Geometry: final body of the model. Coordinates: model frame, mm. A direction names the side the tool comes from. Round coordinates to 2 decimals unless told otherwise and drop trailing zeros. Write each loop counter-clockwise with the first axis right and the second up, starting at its lowest first coordinate (ties: lowest second). Pieces come first, ordered by that corner, then holes.
from build123d import *

# Parameters (mm, degrees)
PAD_DEPTH       = 1.6
SKETCH001_W     = 66
SKETCH001_H     = 48
PAD001_DEPTH    = 26.6
PAD002_DEPTH    = 11.2
SKETCH003_W     = 16
SKETCH003_H     = 8
POCKET_DEPTH    = 16
SKETCH005_R     = 4
SKETCH005_R_2   = 2
PAD003_DEPTH    = 15.6
SKETCH006_W     = 1
SKETCH006_H     = 34.5
SKETCH006_H_2   = 12
PAD004_DEPTH    = 11.6
SKETCH007_R     = 4
SKETCH007_R_2   = 2
PAD005_DEPTH    = 11.6
PAD006_DEPTH    = 24
PAD007_DEPTH    = 66
POCKET002_DEPTH = 0.6
SKETCH018_W     = 48
SKETCH018_H     = 7.5
POCKET003_DEPTH = 2.5
SKETCH008_R     = 1.4
POCKET004_DEPTH = 8


with BuildPart() as part:
    # Sketch → Pad (new body)
    with BuildSketch(Plane.XY):
        with BuildLine():
            Line((-36, 28), (36, 28))
            ThreePointArc((37, 27), (36.707107, 27.707107), (36, 28))
            Line((37, 27), (37, -27))
            ThreePointArc((36, -28), (36.707107, -27.707107), (37, -27))
            Line((36, -28), (-36, -28))
            ThreePointArc((-37, -27), (-36.707107, -27.707107), (-36, -28))
            Line((-37, -27), (-37, 27))
            ThreePointArc((-36, 28), (-36.707107, 27.707107), (-37, 27))
        make_face()
        with BuildLine():
            ThreePointArc((-12.5, 5), (-17.5, 0), (-12.5, -5))
            Line((-12.5, -5), (12.5, -5))
            ThreePointArc((12.5, -5), (17.5, 0), (12.5, 5))
            Line((12.5, 5), (-12.5, 5))
        make_face(mode=Mode.SUBTRACT)
    extrude(amount=PAD_DEPTH)

    # Sketch001 → Pad001 (join)
    with BuildSketch(Plane.XY):
        with BuildLine():
            Line((-36, 28), (36, 28))
            ThreePointArc((37, 27), (36.707107, 27.707107), (36, 28))
            Line((37, 27), (37, -27))
            ThreePointArc((36, -28), (36.707107, -27.707107), (37, -27))
            Line((36, -28), (-36, -28))
            ThreePointArc((-37, -27), (-36.707107, -27.707107), (-36, -28))
            Line((-37, -27), (-37, 27))
            ThreePointArc((-36, 28), (-36.707107, 27.707107), (-37, 27))
        make_face()
        Rectangle(SKETCH001_W, SKETCH001_H, mode=Mode.SUBTRACT)
    extrude(amount=PAD001_DEPTH)

    # Sketch002 → Pad002 (join)
    with BuildSketch(Plane.XY):
        with BuildLine():
            Line((51.5, 9.499999), (38.5, 9.499999))
            ThreePointArc((37, 11.000001), (37.439339, 9.93934), (38.5, 9.499999))
            Line((37, 11.000001), (37, 0))
            Line((37, 0), (37, -11.000001))
            ThreePointArc((38.5, -9.500001), (37.43934, -9.939341), (37, -11.000001))
            Line((38.5, -9.500001), (51.5, -9.500001))
            ThreePointArc((51.5, -9.500001), (52.56066, -9.060661), (53, -8.000001))
            Line((53, 7.999999), (53, -8.000001))
            ThreePointArc((53, 7.999999), (52.56066, 9.060659), (51.5, 9.499999))
        make_face()
    extrude(amount=PAD002_DEPTH)

    # Sketch003 (on DatumPlane) → Pocket (cut)
    with BuildSketch(Plane.YZ.offset(33)):
        with Locations((0, 5.6)):
            Rectangle(SKETCH003_W, SKETCH003_H)
    extrude(amount=POCKET_DEPTH, mode=Mode.SUBTRACT)

    # Sketch005 → Pad003 (join)
    with BuildSketch(Plane.XY):
        with Locations((-11, 15)):
            Circle(SKETCH005_R)
        with Locations((-11, 15)):
            Circle(SKETCH005_R_2, mode=Mode.SUBTRACT)
        with Locations((11, 15)):
            Circle(SKETCH005_R)
        with Locations((11, 15)):
            Circle(SKETCH005_R_2, mode=Mode.SUBTRACT)
    extrude(amount=PAD003_DEPTH)

    # Sketch006 → Pad004 (join)
    with BuildSketch(Plane.XY):
        with Locations((-31, -6.75)):
            Rectangle(SKETCH006_W, SKETCH006_H)
        with Locations((29, -18)):
            Rectangle(SKETCH006_W, SKETCH006_H_2)
    extrude(amount=PAD004_DEPTH)

    # Sketch007 → Pad005 (join)
    with BuildSketch(Plane.XY):
        with Locations((-24, 15)):
            Circle(SKETCH007_R)
        with Locations((-24, 15)):
            Circle(SKETCH007_R_2, mode=Mode.SUBTRACT)
        with Locations((24, 15)):
            Circle(SKETCH007_R)
        with Locations((24, 15)):
            Circle(SKETCH007_R_2, mode=Mode.SUBTRACT)
    extrude(amount=PAD005_DEPTH)

    # Sketch009 → Pad006 (join, symmetric)
    with BuildSketch(Plane.XZ):
        Polygon((-33, 26.6), (-29, 26.6), (-29, 23.6), (-33, 18.832986), align=None)
        Polygon((29, 26.6), (33, 26.6), (33, 18.832986), (29, 23.6), align=None)
    extrude(amount=PAD006_DEPTH, both=True)

    # Sketch010 (on DatumPlane) → Pad007 (join)
    with BuildSketch(Plane(origin=(-33, 0, 0), x_dir=(0, -1, 0), z_dir=(-1, 0, 0))):
        Polygon((-24, 18.832986), (-20, 23.6), (-20, 26.6), (-24, 26.6), align=None)
        Polygon((24, 26.6), (20, 26.6), (20, 23.6), (24, 18.832986), align=None)
    extrude(amount=-PAD007_DEPTH)

    # Sketch011 (on DatumPlane) → Pocket002 (cut)
    with BuildSketch(Plane.XY.offset(26.6)):
        with BuildLine():
            Line((-27.75, 22.25), (27.75, 22.25))
            ThreePointArc((31.25, 18.75), (30.224874, 21.224874), (27.75, 22.25))
            Line((31.25, 18.75), (31.25, -18.75))
            ThreePointArc((27.75, -22.25), (30.224874, -21.224874), (31.25, -18.75))
            Line((27.75, -22.25), (-27.75, -22.25))
            ThreePointArc((-31.25, -18.75), (-30.224874, -21.224874), (-27.75, -22.25))
            Line((-31.25, -18.75), (-31.25, 18.75))
            ThreePointArc((-27.75, 22.25), (-30.224874, 21.224874), (-31.25, 18.75))
        make_face()
        with BuildLine():
            Line((-27.75, 21.25), (27.75, 21.25))
            ThreePointArc((30.25, 18.75), (29.517767, 20.517767), (27.75, 21.25))
            Line((30.25, 18.75), (30.25, -18.75))
            ThreePointArc((27.75, -21.25), (29.517767, -20.517767), (30.25, -18.75))
            Line((27.75, -21.25), (-27.75, -21.25))
            ThreePointArc((-30.25, -18.75), (-29.517767, -20.517767), (-27.75, -21.25))
            Line((-30.25, -18.75), (-30.25, 18.75))
            ThreePointArc((-27.75, 21.25), (-29.517767, 20.517767), (-30.25, 18.75))
        make_face(mode=Mode.SUBTRACT)
    extrude(amount=-POCKET002_DEPTH, mode=Mode.SUBTRACT)

    # Sketch018 (on DatumPlane) → Pocket003 (cut)
    with BuildSketch(Plane(origin=(-33, 0, 0), x_dir=(0, -1, 0), z_dir=(-1, 0, 0))):
        with Locations((0, 5.35)):
            Rectangle(SKETCH018_W, SKETCH018_H)
    extrude(amount=POCKET003_DEPTH, mode=Mode.SUBTRACT)

    # Sketch008 (on DatumPlane) → Pocket004 (cut)
    with BuildSketch(Plane.XY.offset(26.6)):
        with Locations((-34, 25)):
            Circle(SKETCH008_R)
        with Locations((0, 25)):
            Circle(SKETCH008_R)
        with Locations((34, 25)):
            Circle(SKETCH008_R)
        with Locations((-34, -25)):
            Circle(SKETCH008_R)
        with Locations((0, -25)):
            Circle(SKETCH008_R)
        with Locations((34, -25)):
            Circle(SKETCH008_R)
        with Locations((-34, 0)):
            Circle(SKETCH008_R)
        with Locations((34, 0)):
            Circle(SKETCH008_R)
    extrude(amount=-POCKET004_DEPTH, mode=Mode.SUBTRACT)


solid = part.part
1) Line query: probe 1 along Y at (x, z) = (-24, 5); probe 2 along Y at (x, z) = (0, 24.75); probe 3 along X at (y, z) = (-4.5, 5.25). Output: solid intervals per line, ascending.
2) Draft query along Y for faces 1 (the flat face through (37, 0, 13)), 2 (the flat face through (9, 14, 15.6)), 3 (the flat face through (45, 9.5, 6)). Return one class per face: pulls with the +Y half, pulls with the -Y half, needs draft (parallel to the pull), parting line crosses it, or undercut.
3) Reachability of faces 4 (the flat face through (-29.3, -0.1, 26.6)), 5 (the flat face through (0, 20, 25)), 6 (the flat face through (49, 0, 6)) from +Z, -Z, +X, -X, +Y, -Y: full face, straight path, thin tool, end or side. Return the list, or none.
4) Section A-A on z = 4.25. State how many separate pieces and enclosed holes the cut face has, plus the area to 3 significant figures.
5) First-contact query: P1, Ø1.2, axis at x = -34, y = 0, coming from the +Z side; P2, Ø3, axis at x = -25, y = -5.5, coming from the +Z side; P3, Ø4.5, axis at x = 24.5, y = 14, coming from the +Z side. Flat tips, straight axial feed; report the tip coordinate or a pass-through.
6) Section D-D on x = -34. Output: boundary loops of the cut face in (y, z).
Filled in:
1. probe 1: y = -28 to -24, 11 to 13, 17 to 19, 24 to 28
1. probe 2: y = -28 to -26.4, -23.6 to -20, 20 to 23.6, 26.4 to 28
1. probe 3: x = -37 to -35.5, -31.5 to -30.5, 49 to 53
2. face 1: needs draft
2. face 2: undercut
2. face 3: pulls with the +Y half
3. face 4: +Z, +X, -X, +Y, -Y
3. face 5: +Z
3. face 6: none
4. separate pieces: 5
4. enclosed holes: 5
4. area: 1,100 mm2
5. P1: stops at z = 18.6
5. P2: stops at z = 1.6
5. P3: stops at z = 11.6
6. outline: (-28, 0) - (28, 0) - (28, 26.6) - (26.4, 26.6) - (26.4, 18.6) - (23.6, 18.6) - (23.6, 26.6) - (1.4, 26.6) - (1.4, 18.6) - (-1.4, 18.6) - (-1.4, 26.6) - (-23.6, 26.6) - (-23.6, 18.6) - (-26.4, 18.6) - (-26.4, 26.6) - (-28, 26.6) - close; hole (-24, 1.6) - (24, 1.6) - (24, 9.1) - (-24, 9.1) - close
